Autodesk Inventor part; units mm, degrees
ref_plane "YZ Plane" through (0, 0, 0) normal (1, 0, 0) x (0, 1, 0)
ref_plane "XZ Plane" through (0, 0, 0) normal (0, 1, 0) x (-1, 0, 0)
ref_plane "XY Plane" through (0, 0, 0) normal (0, 0, 1) x (1, 0, 0)
sketch "Sketch1" plane through (0, 0, 0) normal (0, 0, 1) x (1, 0, 0)
  line L0 (0, 0) -> (186.538, 0)
  line L1 (186.538, 0) -> (186.538, 60)
  line L2 (186.538, 60) -> (0, 60)
  line L3 (0, 60) -> (0, 0)
  dimension "d0" = 186.538
  dimension "d1" = 60
extrude "Extrusion1" add sketch "Sketch1" along normal blind 6.731
sketch "Sketch2" plane through (0, 0, 6.731) normal (0, 0, 1) x (1, 0, 0)
  line L0 (186.538, 0) -> (186.538, 60)
  line L1 (0, 60) -> (0, 0)
  line L2 (186.538, 40) -> (193.269, 40)
  line L3 (193.269, 40) -> (193.269, 20)
  line L4 (193.269, 20) -> (186.538, 20)
  line L5 (186.538, 20) -> (186.538, 40)
  line L6 (0, 40) -> (-6.731, 40)
  line L7 (-6.731, 40) -> (-6.731, 20)
  line L8 (-6.731, 20) -> (0, 20)
  line L9 (0, 20) -> (0, 40)
  point P0 (0, 30)
  point P1 (0, 30)
  dimension "d4" = 20
  dimension "d5" = 6.731
extrude "Tabs" add sketch "Sketch2" against normal blind 6.731
sketch "Sketch5" plane through (0, 0, 6.731) normal (0, 0, 1) x (1, 0, 0)
  line L0 (193.269, 40) -> (186.538, 40)
  line L1 (0, 40) -> (-6.731, 40)
  line L2 (-6.731, 40) -> (-6.731, 20)
  point P0 (-3.3655, 30)
  point P1 (189.9035, 30)
  point P2 (-6.731, 30)
  point P3 (-6.731, 30)
  point P4 (189.9035, 40)
  point P5 (-3.3655, 40)
hole "TabHole" [suppressed]
sketch "Sketch3" plane through (0, 0, 6.731) normal (0, 0, 1) x (1, 0, 0)
  line L0 (0, 60) -> (0, 40)
  line L1 (-6.731, 40) -> (-6.731, 20)
  line L2 (40, 40) -> (95, 40)
  line L3 (95, 40) -> (95, 20)
  line L4 (95, 20) -> (40, 20)
  line L5 (40, 20) -> (40, 40)
  point P0 (40, 30)
  point P1 (-6.731, 30)
  dimension "d8" = 55
  dimension "d9" = 20
  dimension "d10" = 40
extrude "RibbonHole" cut sketch "Sketch3" against normal up to next
sketch "Sketch4" plane through (0, 0, 6.731) normal (0, 0, 1) x (1, 0, 0)
  line L0 (40, 20) -> (40, 40)
  line L1 (0, 60) -> (0, 40)
  line L2 (0, 20) -> (0, 0)
  line L3 (3, 5.235) -> (3, 54.765) construction
  line L4 (3, 54.765) -> (147.78, 54.765) construction
  point P0 (3, 30)
  point P1 (40, 30)
  point P2 (147.78, 5.235)
  dimension "d13" = 144.78
  dimension "d14" = 49.53
  dimension "d16" = 3
hole "LCDMount" at (3, 54.765, 6.731) at (147.78, 54.765, 6.731) at (147.78, 5.235, 6.731) at (3, 5.235, 6.731) direction (0, 0, -1) diameter 3.176 end through all
sketch "Sketch6" plane through (0, 0, 6.731) normal (0, 0, 1) x (1, 0, 0)
  line L0 (186.538, 60) -> (0, 60)
  line L1 (0, 60) -> (0, 40)
  circle A0 centre (13.5, 45.5) radius 5
  dimension "d31" = 14.5
  dimension "d32" = 13.5
  dimension "d33" = 10
extrude "PotHole" cut sketch "Sketch6" against normal up to next
sketch "Sketch7" plane through (0, 0, 6.731) normal (0, 0, 1) x (1, 0, 0)
  line L0 (-6.731, 20) -> (0, 20)
  line L1 (0, 20) -> (0, 0)
  line L2 (0, 14.088) -> (4.093, 14.088)
  line L3 (4.093, 14.088) -> (4.093, 15.5)
  line L4 (4.093, 15.5) -> (7.269, 15.5)
  line L5 (7.269, 15.5) -> (7.269, 14.088)
  line L6 (7.269, 14.088) -> (11.269, 14.088)
  line L7 (11.269, 14.088) -> (11.269, 10.912)
  line L8 (11.269, 10.912) -> (7.269, 10.912)
  line L9 (7.269, 10.912) -> (7.269, 9.5)
  line L10 (7.269, 9.5) -> (4.093, 9.5)
  line L11 (4.093, 9.5) -> (4.093, 10.912)
  line L12 (4.093, 10.912) -> (0, 10.912)
  line L13 (186.538, 0) -> (186.538, 20)
  line L14 (-6.731, 40) -> (-6.731, 20)
  line L15 (186.538, 14.088) -> (182.445, 14.088)
  line L16 (182.445, 14.088) -> (182.445, 15.5)
  line L17 (182.445, 15.5) -> (179.269, 15.5)
  line L18 (179.269, 15.5) -> (179.269, 14.088)
  line L19 (179.269, 14.088) -> (175.269, 14.088)
  line L20 (175.269, 14.088) -> (175.269, 10.912)
  line L21 (175.269, 10.912) -> (179.269, 10.912)
  line L22 (179.269, 10.912) -> (179.269, 9.5)
  line L23 (179.269, 9.5) -> (182.445, 9.5)
  line L24 (182.445, 9.5) -> (182.445, 10.912)
  line L25 (182.445, 10.912) -> (186.538, 10.912)
  point P0 (11.269, 12.5)
  dimension "d36" = 3.176
  dimension "d38" = 11.269
  dimension "d39" = 4
  dimension "d40" = 6
  dimension "d43" = 7.5
extrude "Nut" cut sketch "Sketch7" against normal up to next
equation "\"d2\" = THICKB"
equation "\"d5\" = THICKB"
equation "\"d6\" = THICKB"
equation "\"THICKA\" = 3.175"
equation "\"THICKB\" = 6.731"
equation "\"THICKC\" = 12.7"
equation "\"THICKPLY\" = 5"
equation "\"MAGDIA\" = 9.5"
equation "\"BALLDIA\" = 12"
properties part number "Controller_Front"
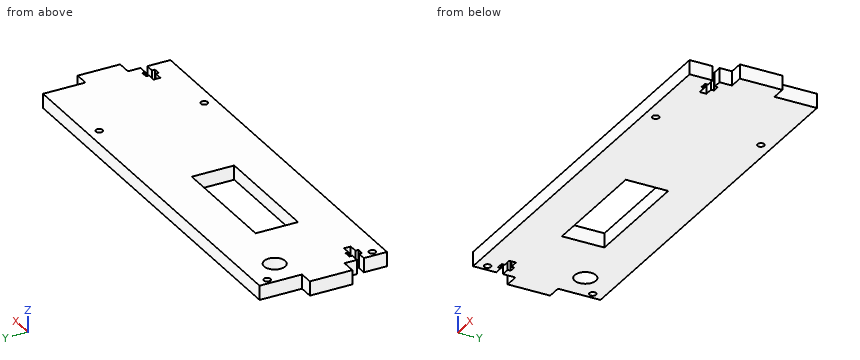
Geometry: final body of the model. Coordinates: model frame, mm. Round coordinates to 2 decimals unless told otherwise and drop trailing zeros. Write each loop counter-clockwise with the first axis right and the second up, starting at its lowest first coordinate (ties: lowest second). Pieces come first, ordered by that corner, then holes. Notation, with made-up numbers: (45, -11) -> (88, -11) arc R16 cw to (88, 18) -> close; hole circle Ø3 at (37, 60). An arc over 180 degrees is marked (long way). Return JSON: item names as keys, results as strings.
Q1. Ray query, line 1 (Y direction, x = 3, z = 2.25); line 2 (Y direction, x = 147.78, z = 2.25); line 3 (Y direction, x = 70, z = 0.5). Return the intervals inside material, ascending.
From the geometry:
{"line 1": "0 to 3.65, 6.82 to 10.91, 14.09 to 53.18, 56.35 to 60", "line 2": "0 to 3.65, 6.82 to 53.18, 56.35 to 60", "line 3": "0 to 20, 40 to 60"}
Q2. Section B-B on y = 28. Return the cut outline in (x, z), and give its area (3 significant figures).
From the geometry:
{"outline": "(-6.73, 0) -> (40, 0) -> (40, 6.73) -> (-6.73, 6.73) -> close; (95, 0) -> (193.27, 0) -> (193.27, 6.73) -> (95, 6.73) -> close", "area": "976 mm2"}
Q3. First-contact query: pin 1 Ø4 at (y, z) = (47.5, 2.5) entering from +X; pin 2 Ø0.7 at (y, z) = (10.5, 3) entering from -X. Flat tips, straight axial feed; report the tip coordinate or a pass-through.
From the geometry:
{"pin 1": "x = 186.54", "pin 2": "x = 0"}
Q4. Section C-C on z = 1.25. Give the number of separate pieces and of enclosed holes in the cut face, and give its area (3 significant figures).
From the geometry:
{"separate pieces": "1", "enclosed holes": "6", "area": "10,200 mm2"}
Q5. Section A-A on x = 13.5. Return the cut outline in (y, z).
From the geometry:
{"outline": "(0, 0) -> (40.5, 0) -> (40.5, 6.73) -> (0, 6.73) -> close; (50.5, 0) -> (60, 0) -> (60, 6.73) -> (50.5, 6.73) -> close"}
